Model file for the job. Use its own axes, mm. A direction names the side the tool comes from. Round coordinates to 2 decimals unless told otherwise and drop trailing zeros. Loops run counter-clockwise (first coordinate to the right, second up) from the corner with the lowest first, then second, coordinate; pieces in that order, holes last. Notation, with made-up numbers: (-2, 52.5) -> (15, 52.5) arc R24 cw to (15, 84.5) -> close; hole circle Ø11 at (-0.75, 35). An arc over 180 degrees is marked (long way). Use a Markdown table: item, result. Add a question column.
```python
from build123d import *

# Parameters (mm, degrees)
SKETCH_2_R           = 32.5
EXTRUDE_2_DEPTH      = 2
SKETCH_3_R           = 2.065299263
SKETCH_3_W           = 3.634517066
SKETCH_3_H           = 0.972738316
SKETCH_3_H_2         = 0.972738315
SKETCH_3_W_2         = 8.575403128
SKETCH_3_H_3         = 0.913568408
SKETCH_3_H_4         = 0.913568407
SKETCH_3_W_3         = 16.93922902
SKETCH_3_H_5         = 2.056372223
SKETCH_3_H_6         = 1.799325695
SKETCH_3_W_4         = 1.799325695
SKETCH_3_H_7         = 8.575403129
SKETCH_3_W_5         = 11.860354008
SKETCH_3_H_8         = 1.369825
SKETCH_3_W_6         = 1.369825
SKETCH_3_H_9         = 11.860354008
CUT_EXTRUDE_1_DEPTH  = 2
EXTRUDE_3_DEPTH      = 7
EXTRUDE_3_DEPTH_BACK = 2
SKETCH_4_R           = 34.00500901
SKETCH_4_R_2         = 32.5
EXTRUDE_START        = 7
EXTRUDE_4_DEPTH      = 7


with BuildPart() as part:
    # 草图2 → 凸台-拉伸2 (new body)
    with BuildSketch(Plane(origin=(0, 0, 0), x_dir=(1, 0, 0), z_dir=(0, 1, 0))):
        with Locations(Location((0, 0, 0), (0, 0, 270))):
            Circle(SKETCH_2_R)
    extrude(amount=EXTRUDE_2_DEPTH)

    # 草图3 → 切除-拉伸1 (cut)
    with BuildSketch(Plane(origin=(0, 2, 0), x_dir=(1, 0, 0), z_dir=(0, 1, 0))):
        with Locations(Location((0.132079869, 0.264159738, 0), (0, 0, 270))):
            Circle(SKETCH_3_R)
        Polygon((4.419781433, 4.838054797), (3.577365341, 4.351685639), (5.394623874, 1.20410153), (6.237039966, 1.690470687), align=None)
        with Locations((0.132079869, 5.777996588)):
            Rectangle(SKETCH_3_W, SKETCH_3_H)
        Polygon((6.237039966, -1.162151211), (5.394623874, -0.675782054), (3.577365341, -3.823366163), (4.419781433, -4.309735321), align=None)
        with Locations((0.132079869, -5.249677113)):
            Rectangle(SKETCH_3_W, SKETCH_3_H_2)
        Polygon((-4.155621695, -4.309735321), (-3.313205603, -3.823366163), (-5.130464136, -0.675782054), (-5.972880228, -1.162151211), align=None)
        Polygon((-5.972880228, 1.690470687), (-5.130464136, 1.20410153), (-3.313205603, 4.351685639), (-4.155621695, 4.838054797), align=None)
        with Locations((0.132079869, 10.044028173)):
            Rectangle(SKETCH_3_W_2, SKETCH_3_H_3)
        Polygon((6.853430322, 9.095744536), (6.062256873, 8.638960332), (10.349958437, 1.212443375), (11.141131886, 1.669227579), align=None)
        Polygon((11.141131886, -1.140908103), (10.349958437, -0.684123899), (6.062256873, -8.110640856), (6.853430322, -8.56742506), align=None)
        with Locations((0.132079869, -9.515708698)):
            Rectangle(SKETCH_3_W_2, SKETCH_3_H_4)
        Polygon((-6.589270584, -8.56742506), (-5.798097135, -8.110640856), (-10.085798699, -0.684123899), (-10.876972148, -1.140908103), align=None)
        Polygon((-10.876972148, 1.669227579), (-10.085798699, 1.212443375), (-5.798097135, 8.638960332), (-6.589270584, 9.095744536), align=None)
        with Locations((0.132079869, 14.903001057)):
            Rectangle(SKETCH_3_W_3, SKETCH_3_H_5)
        Polygon((12.415053578, 13.160619536), (10.459327375, 12.525165572), (15.693837014, -3.584998569), (17.649563217, -2.949544605), align=None)
        Polygon((16.192989615, -7.432417203), (14.984284348, -5.768777127), (1.280160199, -15.725406131), (2.488865465, -17.389046206), align=None)
        Polygon((-2.224705727, -17.389046206), (-1.016000461, -15.725406131), (-14.72012461, -5.768777127), (-15.928829877, -7.432417203), align=None)
        Polygon((-17.385403479, -2.949544605), (-15.429677276, -3.584998569), (-10.195167637, 12.525165572), (-12.15089384, 13.160619536), align=None)
        with Locations((0.132079869, 24.927815646)):
            Rectangle(SKETCH_3_W_2, SKETCH_3_H_6)
        Polygon((9.200480768, 24.546493967), (8.30081792, 22.988232205), (15.727334878, 18.700530641), (16.626997725, 20.258792403), align=None)
        Polygon((20.126712534, 16.759077594), (18.568450772, 15.859414746), (22.856152336, 8.432897789), (24.414414098, 9.332560637), align=None)
        with Locations((24.795735777, 0.264159738)):
            Rectangle(SKETCH_3_W_4, SKETCH_3_H_7)
        Polygon((24.414414098, -8.804241161), (22.856152336, -7.904578313), (18.568450772, -15.331095271), (20.126712534, -16.230758118), align=None)
        Polygon((16.626997725, -19.730472927), (15.727334878, -18.172211165), (8.30081792, -22.459912729), (9.200480768, -24.018174491), align=None)
        with Locations((0.132079869, -24.39949617)):
            Rectangle(SKETCH_3_W_2, SKETCH_3_H_6)
        Polygon((-8.93632103, -24.018174491), (-8.036658182, -22.459912729), (-15.46317514, -18.172211165), (-16.362837987, -19.730472927), align=None)
        Polygon((-19.862552796, -16.230758118), (-18.304291034, -15.331095271), (-22.591992598, -7.904578313), (-24.15025436, -8.804241161), align=None)
        with Locations((-24.531576039, 0.264159738)):
            Rectangle(SKETCH_3_W_4, SKETCH_3_H_7)
        Polygon((-24.15025436, 9.332560637), (-22.591992598, 8.432897789), (-18.304291034, 15.859414746), (-19.862552796, 16.759077594), align=None)
        Polygon((-16.362837987, 20.258792403), (-15.46317514, 18.700530641), (-8.036658182, 22.988232205), (-8.93632103, 24.546493967), align=None)
        Polygon((9.592845567, 18.111462182), (10.561458114, 19.080074729), (18.94799486, 10.693537983), (17.979382313, 9.724925436), align=None)
        with Locations((0.132079869, 20.258792403)):
            Rectangle(SKETCH_3_W_5, SKETCH_3_H_8)
        with Locations((20.126712534, 0.264159738)):
            Rectangle(SKETCH_3_W_6, SKETCH_3_H_9)
        Polygon((17.979382313, -9.19660596), (18.94799486, -10.165218507), (10.561458114, -18.551755253), (9.592845567, -17.583142706), align=None)
        with Locations((0.132079869, -19.730472927)):
            Rectangle(SKETCH_3_W_5, SKETCH_3_H_8)
        Polygon((-9.328685829, -17.583142706), (-10.297298376, -18.551755253), (-18.683835122, -10.165218507), (-17.715222575, -9.19660596), align=None)
        with Locations((-19.862552796, 0.264159738)):
            Rectangle(SKETCH_3_W_6, SKETCH_3_H_9)
        Polygon((-17.715222575, 9.724925436), (-18.683835122, 10.693537983), (-10.297298376, 19.080074729), (-9.328685829, 18.111462182), align=None)
    extrude(amount=-CUT_EXTRUDE_1_DEPTH, mode=Mode.SUBTRACT)

    # 草图4 → 凸台-拉伸3 (add, two sides: drawn at the far end of the back side and taken through both)
    with BuildSketch(Plane(origin=(0, 2, 0), x_dir=(1, 0, 0), z_dir=(0, 1, 0)).offset(-EXTRUDE_3_DEPTH_BACK)):
        with Locations(Location((0, 0, 0), (0, 0, 270))):
            Circle(SKETCH_4_R)
        with Locations(Location((0, 0, 0), (0, 0, 270))):
            Circle(SKETCH_4_R_2, mode=Mode.SUBTRACT)
    extrude(amount=EXTRUDE_3_DEPTH + EXTRUDE_3_DEPTH_BACK)

    # 草图5 → 凸台-拉伸4 (add)
    with BuildSketch(Plane(origin=(0, 0, 0), x_dir=(1, 0, 0), z_dir=(0, 1, 0)).offset(EXTRUDE_START)):
        with BuildLine():
            Line((-34.00500901, 34.00500901), (-104.00500901, 34.00500901))
            Line((-104.00500901, 34.00500901), (-104.00500901, -34.00500901))
            Line((-104.00500901, -34.00500901), (0, -34.00500901))
            ThreePointArc((0, -34.00500901), (-34.00500901, 0), (0, 34.00500901))
            Line((0, 34.00500901), (-34.00500901, 34.00500901))
        make_face()
    extrude(amount=-EXTRUDE_4_DEPTH)


solid = part.part
```
1) Cut at A-A on y = 4.5. Write the cut outline in (x, z) (3 decimals), and give its area (3 significant figures).
2) Cut at B-B on z = 29. Write the cut outline in (x, y) (3 decimals).
3) Pin check, flat tips, straight feed: pin 1 Ø1 at (x, y) = (1.5, 1.5) entering from -Z; pin 2 Ø1.5 at (x, y) = (20, 1.5) entering from +Z; pin 3 Ø3 at (y, z) = (3.5, -22.5) entering from +X. Stop position of each tip, or through.
4) Wall check: probe 1 along X at (y, z) = (6, 1) (3 decimals); probe 2 along Z at (x, y) = (-20, 0.5) (3 decimals); probe 3 along Y at (x, z) = (-6.5, -10.5). Give the ranges that are in metal, low to high. Write a range as from..to.
5) Tool access for faces 1 (the face through (-36, 0, 0)), 2 (the face through (14.696, 1.014, -14.946)), 3 (the face through (9.76, 5.45, 31)): list every direction of +Z, -Z, +X, -X, +Y, -Y with a clear straight run to the whole face (end or side of a thin tool).
6) Pull direction X, two halves, no side cores. Call faces 4 (the face through (33.716, 5.437, -4.427)), 5 (the face through (-9.173, 1.014, 12.341)), 6 (the face through (-104.005, 4, 0)): +X half, -X half, draft (parallel to the pull), parting line (faces both ways), or undercut.
7) Cut at C-C on x = -93. Write the cut outline in (y, z) (3 decimals), and give its area (3 significant figures).
Established:
| question | item | result |
|---|---|---|
| 1 | outline | (-104.005, -34.005) -> (0, -34.005) arc R34.005 ccw to (0, 34.005) -> (-104.005, 34.005) -> close; hole circle Ø65 at (0, 0) |
| 1 | area | 5,570 mm^2 |
| 2 | outline | (-104.005, 0) -> (17.758, 0) -> (17.758, 9) -> (14.671, 9) -> (14.671, 2) -> (-14.671, 2) -> (-14.671, 9) -> (-17.758, 9) -> (-17.758, 7) -> (-104.005, 7) -> close |
| 3 | pin 1 | stops at z = -33.99 |
| 3 | pin 2 | stops at z = 28.03 |
| 3 | pin 3 | stops at x = 26.75 |
| 4 | probe 1 | x = -104.005..-32.485, 32.485..33.99 |
| 4 | probe 2 | z = -34.005..-16.521, -12.922..-6.194, 5.666..12.394, 15.993..34.005 |
| 4 | probe 3 | y = 0..2 |
| 5 | face 1 | +Z, -Z, +X, -X, -Y |
| 5 | face 2 | +Y, -Y |
| 5 | face 3 | +Y |
| 6 | face 4 | parting line |
| 6 | face 5 | undercut |
| 6 | face 6 | -X half |
| 7 | outline | (0, -34.005) -> (7, -34.005) -> (7, 34.005) -> (0, 34.005) -> close |
| 7 | area | 476 mm^2 |
